Input: part model. Units: mm. Frame: model coordinates. Face numbers are marked on the shaded views. A direction names the side the tool comes from. Round coordinates to 2 decimals unless told otherwise and drop trailing zeros. Write each loop counter-clockwise with the first axis right and the second up, starting at its lowest first coordinate (ties: lowest second). Pieces come first, ordered by that corner, then holes. Notation, with made-up numbers: (14, -11.5) -> (49, -11.5) arc R21 cw to (49, 22.5) -> close; hole circle Ø4 at (-29.5, 6.25). An arc over 180 degrees is marked (long way). Use CSV: the item, a comma, the result in double quotes.
```python
from build123d import *

# Parameters (mm, degrees)
SKETCH1_R           = 4.9
SKETCH1_R_2         = 1.9
EXTRUDE_THIN1_DEPTH = 6
CUT_EXTRUDE1_DEPTH  = 2.3


with BuildPart() as part:
    # Sketch1 → Extrude-Thin1 (new body)
    with BuildSketch(Plane(origin=(0, 0, 0), x_dir=(1, 0, 0), z_dir=(0, 1, 0))):
        Circle(SKETCH1_R)
        Circle(SKETCH1_R_2, mode=Mode.SUBTRACT)
    extrude(amount=EXTRUDE_THIN1_DEPTH)

    # Sketch2 → Cut-Extrude1 (cut)
    with BuildSketch(Plane(origin=(0, 6, 0), x_dir=(1, 0, 0), z_dir=(0, 1, 0))):
        Polygon((3.233161507, 0), (1.616580754, 2.8), (-1.616580754, 2.8), (-3.233161507, 0), (-1.616580754, -2.8), (1.616580754, -2.8), align=None)
    extrude(amount=-CUT_EXTRUDE1_DEPTH, mode=Mode.SUBTRACT)


solid = part.part
```
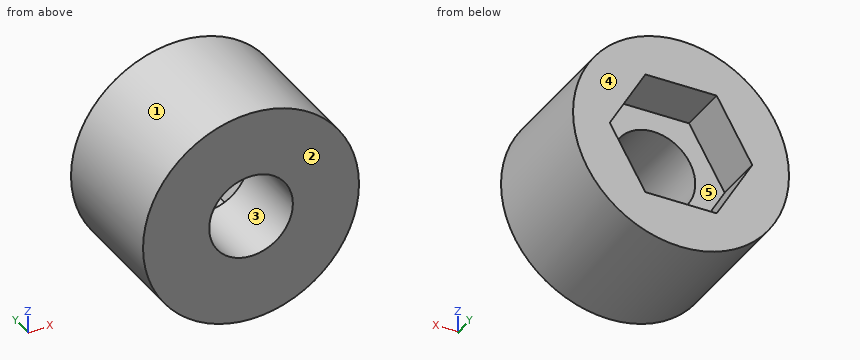
Item 1: Section query D-D on x = 2.5. Return the cut outline in (y, z).
Worked answers:
outline,"(0, -4.21) -> (6, -4.21) -> (6, -1.27) -> (3.7, -1.27) -> (3.7, 1.27) -> (6, 1.27) -> (6, 4.21) -> (0, 4.21) -> close"
Item 2: Section query B-B on z = 1.75. Return the cut outline in (x, y), plus the area to 3 significant figures.
Worked answers:
outline,"(-4.58, 0) -> (-0.74, 0) -> (-0.74, 3.7) -> (-2.22, 3.7) -> (-2.22, 6) -> (-4.58, 6) -> close; (0.74, 0) -> (4.58, 0) -> (4.58, 6) -> (2.22, 6) -> (2.22, 3.7) -> (0.74, 3.7) -> close"
area,"39.2 mm²"
Item 3: Set-up query: the marked faces 4 and 5. Return all of +Z, -Z, +X, -X, +Y, -Y with unobstructed straight access to the full face (end or side cutting, diameter ignored); none if empty.
Worked answers:
face 4,"+Z, -Z, +X, -X, +Y"
face 5,"+Y"
Item 4: Section query A-A on x = 0. Return the cut outline in (y, z), plus the area to 3 significant figures.
Worked answers:
outline,"(0, -4.9) -> (6, -4.9) -> (6, -2.8) -> (3.7, -2.8) -> (3.7, -1.9) -> (0, -1.9) -> close; (0, 1.9) -> (3.7, 1.9) -> (3.7, 2.8) -> (6, 2.8) -> (6, 4.9) -> (0, 4.9) -> close"
area,"31.9 mm²"
Item 5: Pull-direction query (X, two-part tool) for the marked faces 1, 2 and 3; classes: +X half, -X half, draft (parallel to the pull), parting line (faces both ways), or undercut.
Worked answers:
face 1,"parting line"
face 2,"draft"
face 3,"undercut"
Item 6: Line query: line 1 (Z direction, x = 0, y = 1.6); line 2 (Y direction, x = -2.75, z = -0.5). Output: solid intervals per line, ascending.
Worked answers:
line 1,"z = -4.9 to -1.9, 1.9 to 4.9"
line 2,"y = 0 to 3.7"
Item 7: Section query C-C on y = 3.15. Return the cut outline in (x, z).
Worked answers:
outline,"circle Ø9.8 at (0, 0); hole circle Ø3.8 at (0, 0)"
Item 8: First-contact query: pin 1 Ø5 at (x, z) = (0, 0) entering from +Y; pin 2 Ø2 at (y, z) = (2.5, -1.5) entering from +X; pin 3 Ø1 at (y, z) = (4, 2) entering from +X. Flat tips, straight axial feed; report the tip coordinate or a pass-through.
Worked answers:
pin 1,"stops at y = 3.7"
pin 2,"stops at x = 4.87"
pin 3,"stops at x = 4.66"
